from build123d import *

# Parameters (mm, degrees)
F0_R     = 13.9
F1_DEPTH = 16
F2_R     = 15
F2_R_2   = 13.9
F3_DEPTH = 2
F4_R     = 15
F5_DEPTH = 2
F6_R     = 3
F7_DEPTH = 20.001


with BuildPart() as f1:
    # F0 (on Top) → F1 (new body)
    with BuildSketch(Plane.XY):
        Circle(F0_R)
    extrude(amount=F1_DEPTH)

    # F2 (on face) → F3 (join)
    with BuildSketch(Plane.XY.offset(16)):
        Circle(F2_R)
        Circle(F2_R_2, mode=Mode.SUBTRACT)
        Circle(F2_R_2)
    extrude(amount=F3_DEPTH)

    # F4 (on face) → F5 (join)
    with BuildSketch(Plane(origin=(0, 0, 0), x_dir=(1, 0, 0), z_dir=(0, 0, -1))):
        Circle(F4_R)
    extrude(amount=F5_DEPTH)

    # F6 (on face) → F7 (cut, through all)
    with BuildSketch(Plane.XY.offset(18)):
        Circle(F6_R)
    extrude(amount=-F7_DEPTH, mode=Mode.SUBTRACT)


solid = f1.part
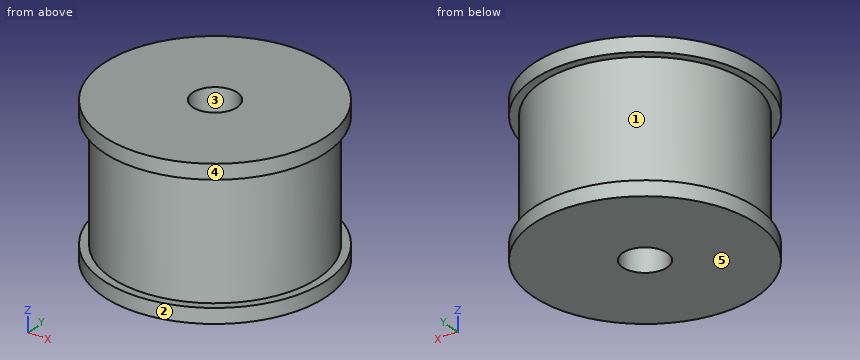
Can you work these out from the model? Positions are in its coordinate system, mm. Face numbers are marked on the shaded views. A direction names the side the tool comes from. Coordinates: 2 decimals unless noted, no trailing zeros. Order: outer loops, then holes, each group sorted by start corner. A loop starts at its lowest first (then second) coordinate and runs counter-clockwise, first axis right, second up. Notation, with made-up numbers: (66.5, -12) - (100.5, -12) arc R27 ccw to (100.5, 23) - close; hole circle Ø10 at (-37, -7). An arc over 180 degrees is marked (long way). Answer as a JSON object with one key per item and string values. Group by question number.
Q1. Imagine slicing it at A-A (x = 0). Please give me the cut outline in (y, z), and give its area (3 significant figures).
Q2. I need wall thicknesses on line 1 (Y direction, x = 0, z = 6.75); line 2 (Z direction, x = 13.25, y = 5.5); line 3 (Y direction, x = -1, z = 11.5). Which ranges of each line are inside material? Lowest first, please. Write a range as from..to.
Q3. On a 3-axis mill with a long thin cutter (end or side, diameter ignored), from which of +Z, -Z, +X, -X, +Y, -Y can I reach the whole of each face in a straight line? I mean the marked faces 1 and 2. Say none if no direction works.
Q4. Imagine slicing it at D-D (z = 1.5). Please give me the cut outline in (x, y), and give its area (3 significant figures).
Q5. Imagine slicing it at C-C (y = -6). Please give me the cut outline in (x, z), and give its area (3 significant figures).
Q6. Will these pins go through, and if not, where does the flat tip stop? P1, Ø1.5, axis at y = -6.5, z = 12, coming from the -X side; P2, Ø10, axis at x = 8.5, z = 2.5, coming from the +Y side; P3, Ø1, axis at x = 5.5, z = 11, coming from the +Y side.
Q7. We'd pull the mould along Y, two halves only. Please class the marked faces 3, 4 and 5: +Y half, -Y half, draft (parallel to the pull), parting line (faces both ways), or undercut.
Determined:
{
 "1": {"outline": "(-15, -2) - (-3, -2) - (-3, 18) - (-15, 18) - (-15, 16) - (-13.9, 16) - (-13.9, 0) - (-15, 0) - close; (3, -2) - (15, -2) - (15, 0) - (13.9, 0) - (13.9, 16) - (15, 16) - (15, 18) - (3, 18) - close", "area": "445 mm2"},
 "2": {"line 1": "y = -13.9..-3, 3..13.9", "line 2": "z = -2..0, 16..18", "line 3": "y = -13.86..-2.83, 2.83..13.86"},
 "3": {"face 1": "none", "face 2": "+Z, -Z"},
 "4": {"outline": "circle Ø27.8 at (0, 0); hole circle Ø6 at (0, 0)", "area": "579 mm2"},
 "5": {"outline": "(-13.75, -2) - (13.75, -2) - (13.75, 0) - (12.54, 0) - (12.54, 16) - (13.75, 16) - (13.75, 18) - (-13.75, 18) - (-13.75, 16) - (-12.54, 16) - (-12.54, 0) - (-13.75, 0) - close", "area": "511 mm2"},
 "6": {"P1": "stops at x = -12.65", "P2": "stops at y = 14.41", "P3": "stops at y = 12.97"},
 "7": {"face 3": "undercut", "face 4": "parting line", "face 5": "draft"}
}
